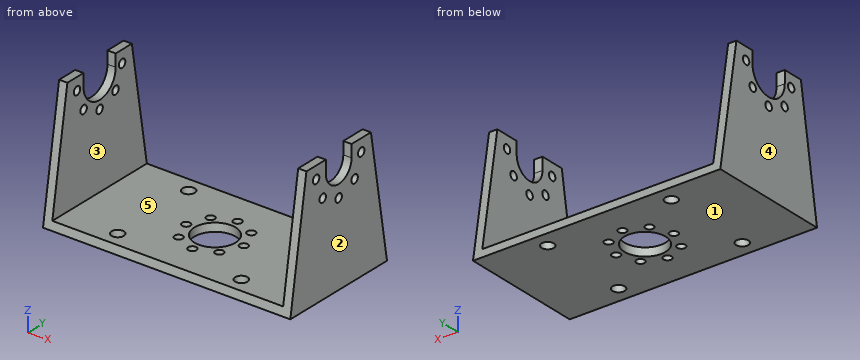
Autodesk Inventor part; units mm, degrees
ref_plane "YZ Plane" through (0, 0, 0) normal (1, 0, 0) x (0, 1, 0)
ref_plane "XZ Plane" through (0, 0, 0) normal (0, 1, 0) x (-1, 0, 0)
ref_plane "XY Plane" through (0, 0, 0) normal (0, 0, 1) x (1, 0, 0)
sketch "スケッチ1" plane through (0, 0, 0) normal (0, 1, 0) x (-1, 0, 0)
  line L0 (30, 14) -> (30, -16)
  line L1 (30, -16) -> (-30, -16)
  line L2 (-30, -16) -> (-30, 14)
  line L3 (28, 14) -> (28, -14)
  line L4 (28, -14) -> (-28, -14)
  line L5 (-28, -14) -> (-28, 14)
  line L6 (-30, 14) -> (-28, 14)
  line L7 (28, 14) -> (30, 14)
  point P0 (0, 0)
  dimension "d0" = 60
  dimension "d2" = 30
  dimension "d3" = 28
  dimension "d4" = 56
  dimension "d5" = 28
  dimension "d6" = 14
  dimension "d7" = 30
  dimension "d8" = 16
  dimension "d9" = 28
  dimension "d11" = 28
extrude "押し出し1" add sketch "スケッチ1" along normal blind 30
sketch "スケッチ2" plane through (30, 0, 14) normal (1, 0, 0) x (0, 0, -1)
  line L0 (30, 0) -> (30, 30)
  line L1 (0, 0) -> (0, 30)
  line L2 (30, 30) -> (0, 25)
  line L3 (30, 0) -> (0, 5)
  point P0 (14, 0)
  dimension "d75" = 20
extrude "押し出し2" cut sketch "スケッチ2" against normal blind 60 keep common part
sketch "スケッチ3" plane through (30, 0, -16) normal (1, 0, 0) x (0, 0, -1)
  line L0 (-30, 5) -> (-30, 25)
  line L1 (0, 0) -> (0, 30)
  arc A0 (-27, 11) -> (-27, 19) centre (-27, 15) ccw
  line L2 (-27, 19) -> (-30, 19)
  line L3 (-27, 11) -> (-30, 11)
  point P0 (-16, 0)
  dimension "d20" = 8
  dimension "d79" = 3
  dimension "d82" = 15
extrude "押し出し3" cut sketch "スケッチ3" against normal blind 2
sketch "スケッチ4" plane through (-30, 0, -16) normal (-1, 0, 0) x (0, 0, 1)
  line L0 (30, 5) -> (30, 25)
  arc A0 (27, 20) -> (27, 10) centre (27, 15) ccw
  line L1 (27, 20) -> (30, 20)
  line L2 (27, 10) -> (30, 10)
  point P0 (16, 0)
  point P1 (0, 30)
  dimension "d25" = 10
  dimension "d80" = 3
  dimension "d81" = 15
extrude "押し出し4" cut sketch "スケッチ4" against normal blind 2
sketch "スケッチ7" plane through (30, 0, -16) normal (0, 0, -1) x (-1, 0, 0)
  line L0 (0, 0) -> (60, 0)
  line L1 (0, 0) -> (0, 30)
  circle A0 centre (30, 15) radius 5
  point P0 (30, 0)
  dimension "d45" = 10
  dimension "d47" = 15
  dimension "d48" = 30
hole "穴2" at (0, 15, -16) direction (0, 0, 1) diameter 10 end through all
sketch "スケッチ8" plane through (30, 0, -16) normal (0, 0, -1) x (-1, 0, 0)
  circle A0 centre (30, 15) radius 5
  line L0 (0, 0) -> (0, 30)
  circle A1 centre (30, 22) radius 1
  line L1 (30, 15) -> (30, 22)
  point P0 (30, 0)
  dimension "d56" = 2
  dimension "d58" = 0
  dimension "d62" = 7
hole "穴3" at (0, 22, -16) direction (0, 0, 1) diameter 2 end through all
pattern_circular "円形状パターン2" count 8 over 360 about axis through (0, 15, 57.4847) along (0, 0, -1) of "穴2", "穴3"
sketch "スケッチ9" plane through (30, 0, -16) normal (1, 0, 0) x (0, 0, -1)
  arc A0 (-27, 11) -> (-27, 19) centre (-27, 15) ccw
  line L0 (-30, 19) -> (-30, 25)
  circle A1 centre (-27, 22) radius 1
  line L1 (-27, 15) -> (-27, 22)
  point P0 (-16, 0)
  dimension "d83" = 2
  dimension "d85" = 7
hole "穴4" at (30, 22, 11) direction (-1, 0, 0) diameter 2 end through all
pattern_circular "円形状パターン3" count 5 over 180 about axis through (30, 15, 11) along (-1, 0, 0) of "穴4"
sketch "スケッチ10" plane through (30, 0, -16) normal (0, 0, -1) x (-1, 0, 0)
  circle A0 centre (30, 15) radius 5
  line L0 (0, 30) -> (60, 30)
  circle A1 centre (15, 26) radius 1.5
  circle A2 centre (15, 4) radius 1.5
  circle A3 centre (45, 4) radius 1.5
  circle A4 centre (45, 26) radius 1.5
  point P0 (30, 0)
  dimension "d96" = 30
  dimension "d98" = 22
  dimension "d99" = 4
  dimension "d100" = 22
  dimension "d101" = 4
  dimension "d102" = 30
  dimension "d103" = 15
  dimension "d104" = 15
  dimension "d105" = 3
hole "穴5" at (15, 4, -16) at (-15, 4, -16) at (-15, 26, -16) at (15, 26, -16) direction (0, 0, 1) diameter 3 end through all
thread "ねじ5"
thread "ねじ6"
thread "ねじ7"
thread "ねじ8"
properties part number "5"
Source: CAD feature listing. Evaluate the final solid. Frame: model axes, mm. Face numbers are marked on the shaded views. A direction names the side the tool comes from. Give positions to 0.01 mm unless a question says otherwise; leave off trailing zeros. Order: outer loops, then holes, each group sorted by start corner. A loop starts at its lowest first (then second) coordinate and runs counter-clockwise, first axis right, second up. Notation, with made-up numbers: (3.5, -4.75) -> (55.5, -4.75) arc R27 ccw to (55.5, 26.25) -> close; hole circle Ø5 at (0, 13.5). An arc over 180 degrees is marked (long way). Use a Markdown table: item, result.
Q1. Section C-C (x = -7). Return the cut outline in (y, z).
A:
| item | result |
|---|---|
| outline | (0, -16) -> (14, -16) -> (14, -14) -> (0.33, -14) -> close; (16, -16) -> (30, -16) -> (29.67, -14) -> (16, -14) -> close |
Q2. First-contact query: P1, Ø6, axis at x = 14.5, y = 4.5, coming from the +Z side; P2, Ø1.6, axis at x = 29.5, z = 12, coming from the -Y side; P3, Ø1, axis at x = 29, z = 12.5, coming from the +Y side. Flat tips, straight axial feed; report the tip coordinate or a pass-through.
A:
| item | result |
|---|---|
| P1 | z = -14 |
| P2 | y = 4.53 |
| P3 | y = 25.33 |
Q3. Section D-D (z = 4). Return the cut outline in (x, y), and give its area (3 significant figures).
A:
| item | result |
|---|---|
| outline | (-30, 3.33) -> (-28, 3.33) -> (-28, 14) -> (-30, 14) -> close; (-30, 16) -> (-28, 16) -> (-28, 26.67) -> (-30, 26.67) -> close; (28, 3.33) -> (30, 3.33) -> (30, 14) -> (28, 14) -> close; (28, 16) -> (30, 16) -> (30, 26.67) -> (28, 26.67) -> close |
| area | 85.3 mm^2 |
Q4. Section A-A (y = 26). Return the cut outline in (x, z), and give its area (3 significant figures).
A:
| item | result |
|---|---|
| outline | (-30, -16) -> (-16.5, -16) -> (-16.5, -14) -> (-28, -14) -> (-28, 8) -> (-30, 8) -> close; (-13.5, -16) -> (13.5, -16) -> (13.5, -14) -> (-13.5, -14) -> close; (16.5, -16) -> (30, -16) -> (30, 8) -> (28, 8) -> (28, -14) -> (16.5, -14) -> close |
| area | 196 mm^2 |
Q5. Material intervals for line 1 (X direction, y = 26, z = -15.05); line 2 (X direction, y = 24.25, z = 12); line 3 (Y direction, x = 29.25, z = 11), sorted ascending. Write a range as [from, to].
A:
| item | result |
|---|---|
| line 1 | [-30, -16.5], [-13.5, 13.5], [16.5, 30] |
| line 2 | [-30, -28], [28, 30] |
| line 3 | [4.5, 7], [9, 11], [19, 21], [23, 25.5] |
Q6. Section B-B (x = 15). Return the cut outline in (y, z).
A:
| item | result |
|---|---|
| outline | (0, -16) -> (2.5, -16) -> (2.5, -14) -> (0.33, -14) -> close; (5.5, -16) -> (24.5, -16) -> (24.5, -14) -> (5.5, -14) -> close; (27.5, -16) -> (30, -16) -> (29.67, -14) -> (27.5, -14) -> close |
Q7. Access query for the marked faces 4 and 5. Directions: +Z, -Z, +X, -X, +Y, -Y. A direction counts if a zero-diameter tool reaches every point of the face in a straight line with its end or side. Return the directions, or none.
A:
| item | result |
|---|---|
| face 4 | +Z, -Z, -X, +Y, -Y |
| face 5 | +Z, +Y, -Y |
Q8. Pull-direction query (X, two-part tool) for the marked faces 1, 2 and 3; classes: +X half, -X half, draft (parallel to the pull), parting line (faces both ways), or undercut.
A:
| item | result |
|---|---|
| face 1 | draft |
| face 2 | +X half |
| face 3 | undercut |
